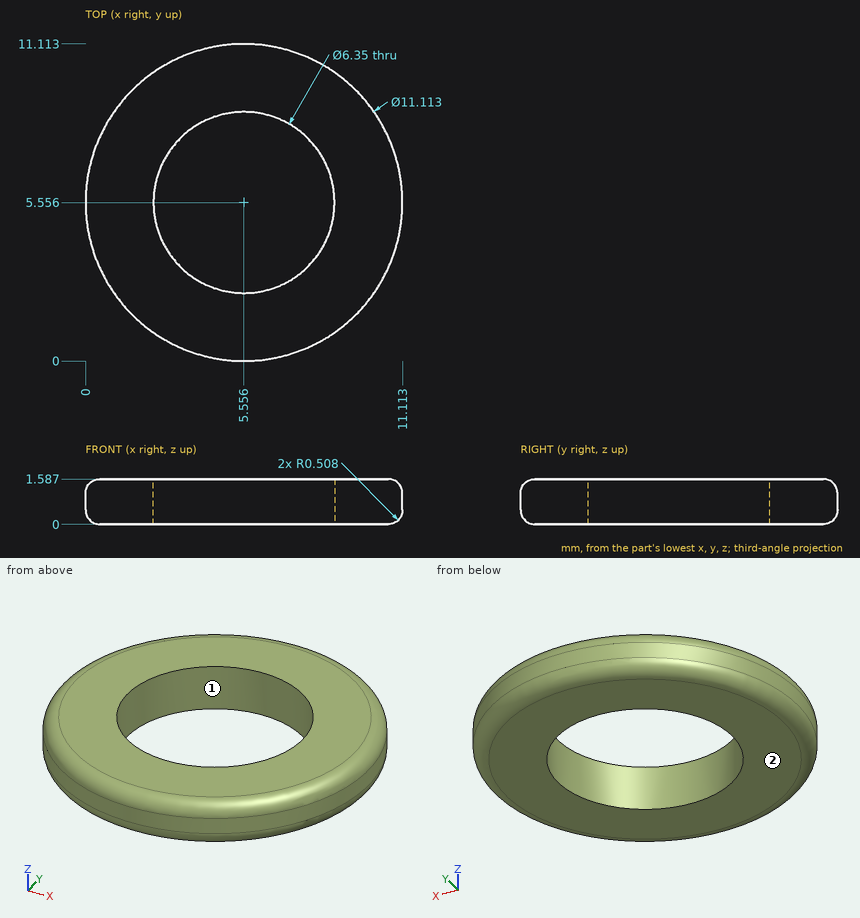
Design review of the part shown in the three views and the two pictorial views. Dimensions are in mm from the part's minimum x, y and z. Give positions to 0.01 mm unless a question says otherwise; leave off trailing zeros. Answer in a Markdown table with one row per item.
1) Mouldability with a two-part tool opening along Y and no side actions: class the marked faces 1 and 2 as +Y half, -Y half, draft (parallel to the pull), parting line (faces both ways), or undercut.
Worked answers:
| item | result |
|---|---|
| face 1 | undercut |
| face 2 | draft |
2) Clearance check with a flat-ended pin moving along its axis: P1, Ø5.5, axis at x = 5.56, y = 5.56, coming from the -Z side. State where the tip first meets the part, or that it passes through.
Worked answers:
| item | result |
|---|---|
| P1 | through |
3) For L1, parallel to Y at x = 5.25, z = 1.05 (1 decimal); L2, parallel to X at y = 5.75, z = 0.2 (1 decimal); L3, parallel to X at y = 3.75, z = 1.05 (1 decimal), list the stretches that pass through material, from the lowest coordinate up. Write a range as [from, to].
Worked answers:
| item | result |
|---|---|
| L1 | [0, 2.4], [8.7, 11.1] |
| L2 | [0.1, 2.4], [8.7, 11] |
| L3 | [0.3, 2.9], [8.2, 10.8] |
